Verification items for the finished model (mm, model axes). A direction names the side the tool comes from. Coordinates: 2 decimals unless noted, no trailing zeros. Order: outer loops, then holes, each group sorted by start corner. A loop starts at its lowest first (then second) coordinate and runs counter-clockwise, first axis right, second up. Notation, with made-up numbers: (5.5, 14.5) -> (38.5, 14.5) arc R32 ccw to (38.5, 50.5) -> close; hole circle Ø3 at (37, 33). An arc over 180 degrees is marked (long way). Answer as CSV lines item,"result".
Autodesk Inventor part; units mm, degrees
ref_plane "YZ Plane" through (0, 0, 0) normal (1, 0, 0) x (0, 1, 0)
ref_plane "XZ Plane" through (0, 0, 0) normal (0, 1, 0) x (-1, 0, 0)
ref_plane "XY Plane" through (0, 0, 0) normal (0, 0, 1) x (1, 0, 0)
sketch "Sketch1" plane through (0, 0, 0) normal (0, 1, 0) x (-1, 0, 0)
  line L0 (0, 0) -> (41.5, 0)
  line L1 (41.5, 0) -> (2.6101, 40.0152)
  line L2 (2.6101, 40.0152) -> (0, 0)
  line L3 (-38.7898, 77.591) -> (-33.77, 82.4696)
  line L4 (-33.77, 82.4696) -> (44.0099, 2.4393)
  line L5 (44.0099, 2.4393) -> (38.9901, -2.4393)
  line L6 (38.9901, -2.4393) -> (-38.7898, 77.591)
  line L7 (-38.7898, 77.591) -> (44.0099, 2.4393) construction
  line L8 (-33.77, 82.4696) -> (38.9901, -2.4393) construction
  line L9 (83, -3.5) -> (83, 3.5)
  line L10 (83, 3.5) -> (0, 3.5)
  line L11 (0, 3.5) -> (0, -3.5)
  line L12 (0, -3.5) -> (83, -3.5)
  line L13 (83, -3.5) -> (0, 3.5) construction
  line L14 (83, 3.5) -> (0, -3.5) construction
  line L15 (-6.1026, -39.7873) -> (0.8825, -40.243)
  line L16 (0.8825, -40.243) -> (6.1026, 39.7873)
  line L17 (6.1026, 39.7873) -> (-0.8825, 40.243)
  line L18 (-0.8825, 40.243) -> (-6.1026, -39.7873)
  line L19 (-6.1026, -39.7873) -> (6.1026, 39.7873) construction
  line L20 (0.8825, -40.243) -> (-0.8825, 40.243) construction
  circle A0 centre (0, 0) radius 1.65
  circle A1 centre (2.6101, 40.0152) radius 1.65
  circle A2 centre (41.5, 0) radius 1.65
  line L21 (2.6101, 40.0152) -> (-2.6009, 40.355)
  line L22 (-1.2742, 34.2377) -> (-0.3698, 48.1031)
  line L23 (-0.3698, 48.1031) -> (-5.0836, 42.9096)
  line L24 (-2.6009, 40.355) -> (2.1129, 45.5486)
  line L25 (6.5967, -3.5) -> (-3.7357, -3.5)
  line L26 (10.4211, 3.5) -> (-3.2791, 3.5)
  line L27 (44.9726, 3.5) -> (44.9726, -3.5731)
  point P0 (33.2178, 3.5)
  point P1 (3.7357, 3.5)
  point P2 (5.5899, 31.9272)
  point P3 (42.9791, 3.5)
  point P4 (-0.7416, 42.4036)
  point P5 (44.9726, -3.5)
  dimension "d0" = 41.5
  dimension "d1" = 55.8
  dimension "d2" = 45.817
  dimension "d3" = 7
  dimension "d4" = 7
  dimension "d5" = 7
  dimension "d6" = 3.3
  dimension "d7" = 3.3
  dimension "d8" = 3.3
extrude "Extrusion1" add sketch "Sketch1" along normal blind 5 contours A0 L2 L10 L16 L0 | L0 L16 L12 L11 A0 | A0 L11 L10 L2 | A0 L11 L25 L18 L26 | L16 L10 L6 L0 | L0 L6 L5 A2 L4 L10 L27 L12 L16 | L10 L26 L18 L6 L2 | L2 L6 L16 L10 | L6 L10 L1 A2 L0 | L0 A2 L5 L6 | L6 L18 L17 A1 L2 | L2 A1 L1 L16 L6 | L6 L16 L1 L10 | L1 L10 L4 L5 A2 | L1 L16 L17 A1 L22 L24 L4 L10 | L1 A1 L17 L16
sketch "Sketch2" plane through (0, 5, 0) normal (0, 1, 0) x (1, 0, 0)
  line L0 (-42.9791, -3.5) -> (-2.1129, -45.5486)
  line L1 (-41.9322, -4.5771) -> (-44.9726, -1.4485)
  line L2 (-44.9726, 3.5) -> (-44.9726, -3.5)
  line L3 (-41.9322, -4.5771) -> (-37.5696, -4.5771) construction
  line L4 (-44.9726, -1.4485) -> (-44.9726, -3.5)
  line L5 (-44.9726, -3.5) -> (-42.9791, -3.5)
  point P0 (0, 0)
  dimension "d11" = 134.18
extrude "Extrusion2" cut sketch "Sketch2" against normal blind 10
sketch "Sketch3" plane through (0, 5, 0) normal (0, 1, 0) x (1, 0, 0)
  line L0 (-44.9726, -1.4485) -> (-41.9322, -4.5771)
  line L1 (-44.9726, 3.5) -> (-44.9726, -1.4485)
  line L2 (-44.9726, -1.4485) -> (-44.9726, 3.5)
  line L3 (-44.9726, 3.5) -> (-53.5355, 3.5)
  line L4 (-41.9322, -4.5771) -> (-49.7814, 3.5)
  line L5 (-41.9322, -4.5771) -> (-2.1129, -45.5486)
  line L6 (-6.7195, -40.8087) -> (1.7936, -49.5681)
  line L7 (0.7416, -42.4036) -> (3.7357, 3.5)
  line L8 (0.9497, -39.2136) -> (0.3698, -48.1031)
  line L9 (-2.1129, -45.5486) -> (0.7416, -42.4036)
  line L10 (-2.1129, -45.5486) -> (0.7416, -42.4036)
  point P0 (0, 0)
extrude "Extrusion3" add sketch "Sketch3" against normal blind 5
fillet "Fillet1" radius 3 3 edges at (0.3698, 2.5, 48.1031) (-49.7814, 2.5, -3.5) (3.7357, 2.5, -3.5)
properties part number "bde"
Item 1: Section check C-C, the plane y = 3.6. Count the separate pieces of the cut face and the enclosed holes in it, plus the area to 3 significant figures.
Answer list:
separate pieces,"1"
enclosed holes,"4"
area,"913 mm2"
Item 2: Tool access check on faces 1 (the flat face through (-4.65, 2.46, 17.51)), 2 (the flat face through (-21, 2, -3.5)). Record the directions out of +Z, -Z, +X, -X, +Y, -Y that give a thin tool (end or side, any length) a straight path to the whole face; none if there is none.
Answer list:
face 1,"+Y, -Y"
face 2,"-Z, +X, -X, +Y, -Y"
Item 3: Depth check by flat-ended pin: pin 1 Ø1.5 at (x, y) = (-9, 4) entering from +Z; pin 2 Ø1.5 at (x, z) = (-28.5, 14.5) entering from -Y; pin 3 Ø1.5 at (x, y) = (-12.5, 1.5) entering from +Z; pin 4 Ø1 at (x, y) = (-5.5, 2) entering from +Z. Enter the tip coordinate at first touch or a pass-through.
Answer list:
pin 1,"z = 39.23"
pin 2,"y = 0"
pin 3,"z = 35.63"
pin 4,"z = 42.58"
Item 4: Section check D-D, the plane z = 33. Record the boundary of the cut face in (x, y), plus the area to 3 significant figures.
Answer list:
outline,"(-14.31, 0) -> (1.35, 0) -> (1.35, 5) -> (-14.31, 5) -> close"
area,"78.3 mm2"
Item 5: Section check B-B, the plane x = -41.5. Record the boundary of the cut face in (y, z).
Answer list:
outline,"(0, -3.5) -> (5, -3.5) -> (5, -1.65) -> (0, -1.65) -> close; (0, 1.65) -> (5, 1.65) -> (5, 5.02) -> (0, 5.02) -> close"
Item 6: Section check A-A, the plane z = 9. Record the boundary of the cut face in (x, y).
Answer list:
outline,"(-37.63, 0) -> (-27.87, 0) -> (-27.87, 5) -> (-37.63, 5) -> close; (-4.09, 0) -> (2.92, 0) -> (2.92, 5) -> (-4.09, 5) -> close"
Item 7: Release check for a two-part mould opening along X. For faces 3 (the flat face through (-19.6, 2.46, 17.51)), 4 (the cylindrical face through (2.746, 2.535, -2.526)), 5 (the flat face through (-16, 5, 22)) record: +X half, -X half, draft (parallel to the pull), parting line (faces both ways), or undercut.
Answer list:
face 3,"undercut"
face 4,"+X half"
face 5,"draft"
Item 8: Thickness scan on line 1 (X direction, y = 1.8, z = 0); line 2 (Z direction, x = -24, y = 3.8); line 3 (Z direction, x = 0, y = 3.5). Record the ranges inside material, lowest first.
Answer list:
line 1,"-45.64 to -43.15, -39.85 to -1.65, 1.65 to 3.51"
line 2,"-3.5 to 3.5, 12.98 to 23.03"
line 3,"-3.5 to -1.65, 1.65 to 43.23"
